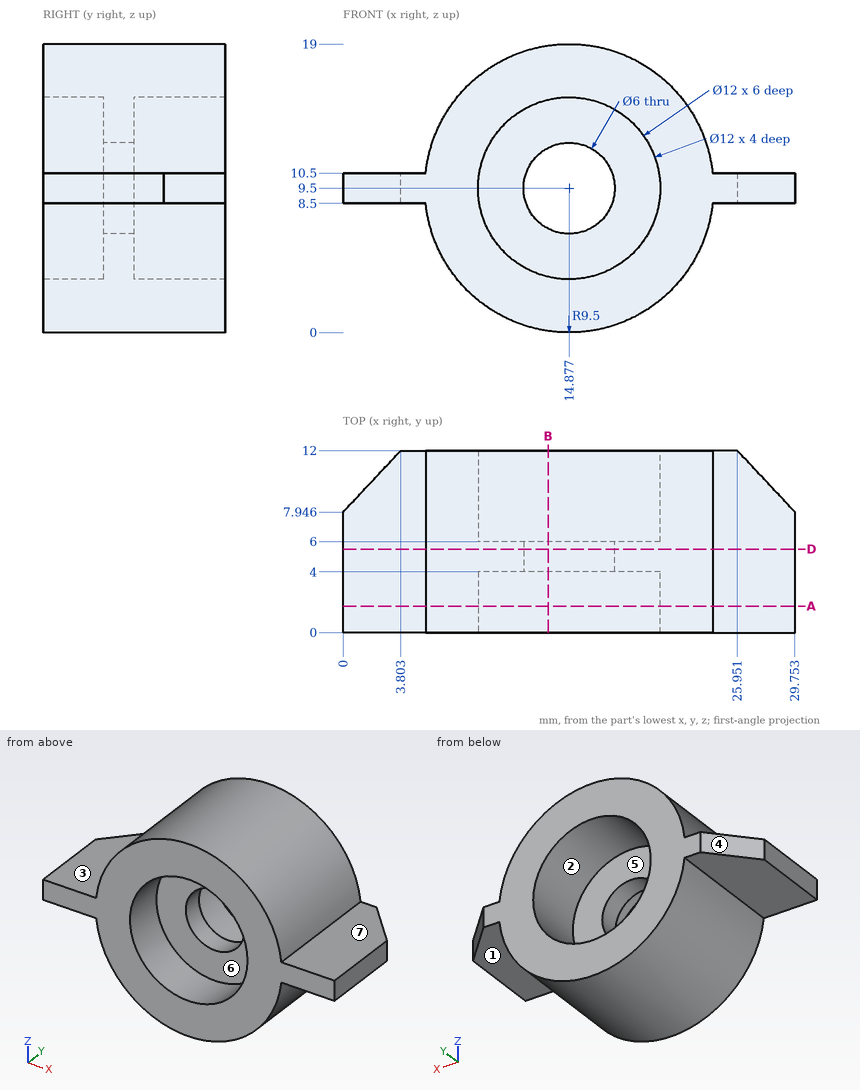
Geometry: see drawing. Coordinates: mm, zero at the bounding-box minimum. A direction names the side the tool comes from. Coordinates: 2 decimals unless noted, no trailing zeros. Write each loop counter-clockwise with the first axis right and the second up, starting at its lowest first coordinate (ties: lowest second). Pieces come first, ordered by that corner, then holes.
1) Section D-D on y = 5.5. Output: boundary loops of the cut face in (x, z), and give its area (3 significant figures).
2) Material intervals for line 1 along X through (y, z) = (5.45, 9.5); line 2 along X through (y, z) = (1.8, 9.5); line 3 along Z through (x, y) = (4.5, 9), sorted ascending.
3) Section A-A on y = 1.75. Output: boundary loops of the cut face in (x, z).
4) Pin query (flat end, axial travel): pin 1 Ø6 at (x, y) = (4.5, 4) entering from +Z (1 decimal); pin 2 Ø4 at (y, z) = (8, 13.5) entering from -X; pin 3 Ø6 at (x, y) = (26, 7.5) entering from +Z (1 decimal). Return the tip coordinate at first contact, or that it passes through.
5) Section B-B on x = 13.5. Output: boundary loops of the cut face in (y, z) (1 decimal).
6) Set-up query: the marked faces 1, 2 and 3. Return all of +Z, -Z, +X, -X, +Y, -Y with unobstructed straight access to the full face (end or side cutting, diameter ignored); none if empty.
7) Mould query, pull axis X, two halves, no side actions, for the marked faces 4, 5, 6 and 7. Classes: pulls with the +X half, pulls with the -X half, needs draft (parallel to the pull), parting line crosses it, or undercut.
Check result:
1. outline: (0, 8.5) - (5.43, 8.5) arc R9.5 ccw to (24.32, 8.5) - (29.75, 8.5) - (29.75, 10.5) - (24.32, 10.5) arc R9.5 ccw to (5.43, 10.5) - (0, 10.5) - close; hole circle Ø6 at (14.88, 9.5)
1. area: 277 mm2
2. line 1: x = 0 to 11.88, 17.88 to 29.75
2. line 2: x = 0 to 8.88, 20.88 to 29.75
2. line 3: z = 8.5 to 10.5
3. outline: (0, 8.5) - (5.43, 8.5) arc R9.5 ccw to (24.32, 8.5) - (29.75, 8.5) - (29.75, 10.5) - (24.32, 10.5) arc R9.5 ccw to (5.43, 10.5) - (0, 10.5) - close; hole circle Ø12 at (14.88, 9.5)
4. pin 1: stops at z = 15.5
4. pin 2: stops at x = 5.59
4. pin 3: stops at z = 14.4
5. outline: (0, 0.1) - (12, 0.1) - (12, 3.7) - (6, 3.7) - (6, 6.8) - (4, 6.8) - (4, 3.7) - (0, 3.7) - close; (0, 15.3) - (4, 15.3) - (4, 12.2) - (6, 12.2) - (6, 15.3) - (12, 15.3) - (12, 18.9) - (0, 18.9) - close
6. face 1: -Z, +X, +Y, -Y
6. face 2: +Y
6. face 3: +Z, -X, +Y, -Y
7. face 4: pulls with the -X half
7. face 5: undercut
7. face 6: undercut
7. face 7: needs draft
